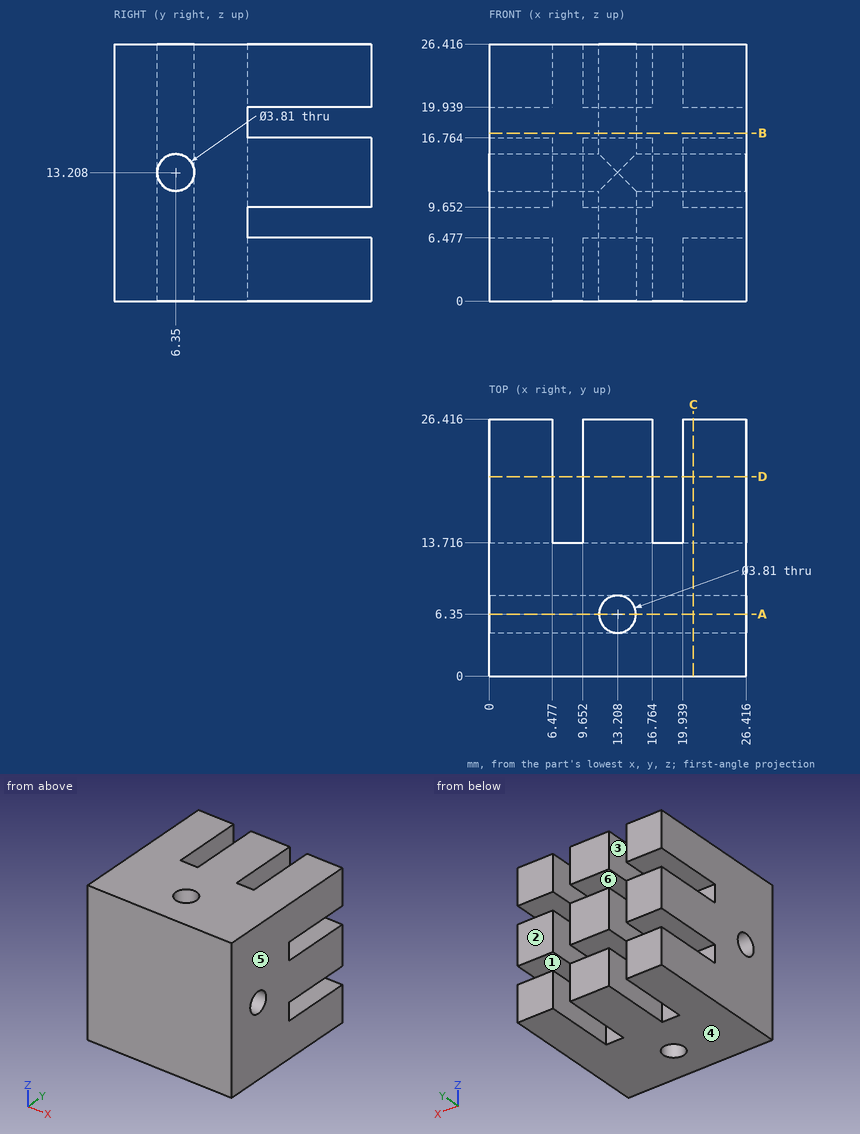
For this review, use the dimensioned drawing (mm, ordinates from the lowest corner) and the shaded views. A direction names the side the tool comes from. Round coordinates to 2 decimals unless told otherwise and drop trailing zeros. Order: outer loops, then holes, each group sorted by start corner. A loop starts at its lowest first (then second) coordinate and runs counter-clockwise, first axis right, second up. Notation, with made-up numbers: (-3.75, 18) - (32.25, 18) arc R18 cw to (32.25, 23) - close; hole circle Ø6 at (-29, -34.5). An arc over 180 degrees is marked (long way). Use one line per item in the form item = value.
Q1. Add section A-A on y = 6.35. Give the boundary of the cut face in (x, z), then the cut area to 3 significant figures.
Response values:
outline = (0, 0) - (11.3, 0) - (11.3, 11.3) - (0, 11.3) - close; (0, 15.11) - (11.3, 15.11) - (11.3, 26.42) - (0, 26.42) - close; (15.11, 0) - (26.42, 0) - (26.42, 11.3) - (15.11, 11.3) - close; (15.11, 15.11) - (26.42, 15.11) - (26.42, 26.42) - (15.11, 26.42) - close
area = 511 mm^2
Q2. Clearance check with flat-ended pins moving along their axes: P1, Ø1.9, axis at x = 22.5, y = 20.5, coming from the -Z side; P2, Ø3.5, axis at y = 6.35, z = 13.208, coming from the +X side. State where each tip first meets the part, or that it passes through.
Response values:
P1 = 0
P2 = through
Q3. Mouldability with a two-part tool opening along Z and no side actions: class the marked faces 4, 5 and 6 as pulls with the +Z half, pulls with the -Z half, needs draft (parallel to the pull), parting line crosses it, or undercut.
Response values:
face_4 = pulls with the -Z half
face_5 = needs draft
face_6 = undercut
Q4. Add section D-D on y = 20.5. Give the number of separate pieces and of enclosed holes in the cut face, then the cut area to 3 significant figures.
Response values:
separate_pieces = 9
enclosed_holes = 0
area = 403 mm^2
Q5. Add section B-B on z = 17.25. Give the boundary of the cut face in (x, y) (3 decimals), then the cut area to 3 significant figures.
Response values:
outline = (0, 0) - (26.416, 0) - (26.416, 13.716) - (0, 13.716) - close; hole circle Ø3.81 at (13.208, 6.35)
area = 351 mm^2
Q6. Tool access review of the marked faces 1, 2 and 3: name each direction out of +Z, -Z, +X, -X, +Y, -Y from which nothing blocks a thin tool from reaching the whole face with its end or side.
Response values:
face_1 = +X, -X, +Y
face_2 = +Z, -Z, +X, -X, +Y
face_3 = +Z, -Z, +Y
Q7. To check wall thickness, follow line 1 (Z direction, x = 25.5, y = 20.5); line 2 (Z direction, x = 6.5, y = 6.35). State the ranges of each line that lie inside material, in increasing order.
Response values:
line_1 = 0 to 6.48, 9.65 to 16.76, 19.94 to 26.42
line_2 = 0 to 11.3, 15.11 to 26.42
Q8. Add section C-C on x = 21. Give the boundary of the cut face in (y, z) (3 decimals).
Response values:
outline = (0, 0) - (26.416, 0) - (26.416, 6.477) - (13.716, 6.477) - (13.716, 9.652) - (26.416, 9.652) - (26.416, 16.764) - (13.716, 16.764) - (13.716, 19.939) - (26.416, 19.939) - (26.416, 26.416) - (0, 26.416) - close; hole circle Ø3.81 at (6.35, 13.208)
